Geometry: final body of the model. Coordinates: model frame, mm. A direction names the side the tool comes from. Coordinates: 2 decimals unless noted, no trailing zeros. Write each loop counter-clockwise with the first axis right and the second up, starting at its lowest first coordinate (ties: lowest second). Pieces come first, ordered by that corner, then holes. Notation, with made-up numbers: (27.5, 89) -> (59.5, 89) arc R24 ccw to (59.5, 103) -> close; hole circle Ø1 at (20, 72). An arc over 180 degrees is marked (long way). Answer as a JSON object with one key per item and string values. Group by question number.
Autodesk Inventor part; units mm, degrees
ref_plane "Work Plane1" through (1.525, 0, 0) normal (0, 0, 1) x (1, 0, 0)
ref_plane "YZ Plane" through (0, 0, 0) normal (1, 0, 0) x (0, 1, 0)
ref_plane "XZ Plane" through (0, 0, 0) normal (0, 1, 0) x (-1, 0, 0)
sketch "Sketch1" plane through (0, 0, 0) normal (0, 0, 1) x (1, 0, 0)
  line L0 (0, 7.315) -> (0, 5)
  line L1 (4.5, 5) -> (25, 5)
  line L2 (25, 5) -> (25, 0)
  line L3 (25, 0) -> (-0.6001, 0)
  line L4 (-5.7201, 0) -> (30.12, 0)
  line L5 (-0.6001, 0) -> (-0.6001, 7.315)
  line L6 (-0.6001, 7.315) -> (0, 7.315)
  line L7 (4.5, 5) -> (3.5797, 5)
  line L8 (3.5797, 5) -> (0, 5)
  line L9 (0, -1.463) -> (0, 8.778)
  dimension "d0" = 25
  dimension "d1" = 20.5
  dimension "d2" = 10
  dimension "d9" = 0.6001
  dimension "d10" = 14.63
  dimension "d13" = 0.9203
  dimension "d14" = 10
revolve "Body" add sketch "Sketch1" angle 360 about axis through (25, 0, 0) along (-1, 0, 0)
sketch "Sketch2" plane through (-0.6001, 0, 0) normal (-1, 0, 0) x (0, 0, 1)
  line L0 (0, 9.2376) -> (8, 4.6188)
  line L1 (8, 4.6188) -> (8, -4.6188)
  line L2 (8, -4.6188) -> (0, -9.2376)
  line L3 (0, -9.2376) -> (-8, -4.6188)
  line L4 (-8, -4.6188) -> (-8, 4.6188)
  line L5 (-8, 4.6188) -> (0, 9.2376)
  point P0 (0, 0)
  point P1 (0, 0)
  dimension "d11" = 16
extrude "Head" add sketch "Sketch2" along normal blind 5.8
sketch "Sketch4" plane through (0, 0, 0) normal (0, 0, 1) x (1, 0, 0)
  line L0 (-6.4001, 8) -> (-6.4001, 9.2376)
  line L1 (-6.4001, 9.2376) -> (-5.6856, 9.2376)
  line L2 (-5.6856, 9.2376) -> (-6.4001, 8)
  line L3 (-7.5601, 0) -> (0.5599, 0)
  line L4 (-0.6001, 9.2376) -> (-6.4001, 9.2376)
  line L5 (-6.4001, 4.6188) -> (-6.4001, 9.2376)
  dimension "d5" = 30
  dimension "d19" = 16
revolve "Chamfer1" cut sketch "Sketch4" angle 360 about axis through (-10, 0, 0) along (1, 0, 0)
thread "Thread"
chamfer "Chamfer2" distance 0.9202 distance2 0.9203 1 edges at (25, -5, 0) measured on face at (25, 1.974, 0.2121)
ref_plane "Work Plane1" through (1.525, 0, 0) normal (0, 0, 1) x (1, 0, 0)
equation "\"d11\" = SW"
equation "\"d3\" = KOH - SD"
equation "\"d15\" = GEL"
equation "\"d6\" = -0.5 * SPD + 0.5 * GD"
equation "\"d0\" = NLG"
equation "\"d1\" = GEL"
equation "\"d2\" = GD"
equation "\"d10\" = SD2"
equation "\"d14\" = BDM"
equation "\"d5\" = ANG1"
equation "\"d19\" = SW0"
equation "\"NLG\" = 25"
equation "\"GD\" = NND"
equation "\"BDM\" = NND"
equation "\"KOH\" = 6.4"
equation "\"GEL\" = 20.5"
equation "\"SW\" = 16"
equation "\"SW0\" = SW"
equation "\"SPD\" = NND - 1.2269 * PTC"
equation "\"SD2\" = 14.63"
equation "\"SD\" = 0.6"
equation "\"ANG1\" = 30deg"
equation "\"GAL\" = 0.61345 * PTC"
equation "\"GUL\" = 0.61345 * PTC"
equation "\"RR\" = 0.4"
equation "\"GD1\" = THREADDIA - 1.2269 * PTC"
equation "\"SDH\" = SD2"
equation "\"SDHG\" = 4.5"
equation "\"TOA\" = 30deg"
equation "\"PTC\" = 1.5"
equation "\"E0\" = 18.48"
properties part number "ISO 4017 - M10 x 25" material "Steel, Mild"
Item 1: Contact query for flat-ended pins moving along their axis: pin 1 (2 mm diameter, centred on x = 15.5, z = 2.5, fed in from -Y); pin 2 (4 mm diameter, centred on x = -3, z = -4.5, fed in from -Y); pin 3 (8 mm diameter, centred on y = -3.5, z = -3, fed in from +X); pin 4 (1.5 mm diameter, centred on y = 4.5, z = 6, fed in from +X). Output: stop coordinate, or through.
Item 2: Section A-A on x = -1.5. Output: boundary loops of the cut face in (y, z), then the cut area to 3 significant figures.
Item 3: Set-up query: faces 1 (the conical face through (-6.226, -4.168, -7.179)), 2 (the cylindrical face through (11.87, -1.08, 4.88)). Return all of +Z, -Z, +X, -X, +Y, -Y with unobstructed straight access to the full face (end or side cutting, diameter ignored); none if empty.
Item 4: Section B-B on x = 20.5. Output: boundary loops of the cut face in (y, z).
Item 5: Ray query, L1, parallel to X at y = -8, z = -0.25; L2, parallel to X at y = 3.75, z = 5.5; L3, parallel to Z at x = 17.5, y = 3. Return the intervals inside material, ascending. Write a range as [from, to].
Answer sheet:
{
 "1": {"pin 1": "stops at y = -4.77", "pin 2": "stops at y = -7.79", "pin 3": "stops at x = 25", "pin 4": "stops at x = 0"},
 "2": {"outline": "(-9.24, 0) -> (-4.62, -8) -> (4.62, -8) -> (9.24, 0) -> (4.62, 8) -> (-4.62, 8) -> close", "area": "222 mm^2"},
 "3": {"face 1": "-Z, -X, -Y", "face 2": "+X"},
 "4": {"outline": "circle Ø10 at (0, 0)"},
 "5": {"L1": "x = [-6.4, -0.6]", "L2": "x = [-6.4, 0]", "L3": "z = [-4, 4]"}
}
